The model under review builds one solid part; all positions refer to its coordinate system, in mm. A direction names the side the tool comes from. Round coordinates to 2 decimals unless told otherwise and drop trailing zeros. Write each loop counter-clockwise with the first axis right and the second up, starting at its lowest first coordinate (ties: lowest second). Pieces come first, ordered by that corner, then holes. Notation, with made-up numbers: (74.25, 74.25) -> (124.25, 74.25) arc R8 cw to (124.25, 82.25) -> close; hole circle Ø5 at (-2, 57). An arc over 180 degrees is marked (long way). Return JSON: item names as keys, results as strings. Group by question number.
1. Take a section at D-D, the plane y = -10. Write out the cut boundary in (x, z), then the cut area to 3 significant figures.
2. Take a section at A-A, the plane y = 18. Write out the cut boundary in (x, z), then the cut area to 3 significant figures.
3. For line 1 along Y through (x, z) = (-51.5, 8); line 2 along Y through (x, z) = (-27.5, 22); line 3 along X through (y, z) = (-12, 22), list the stretches that pass through material, from the lowest coordinate up. Write a range as from..to.
4. Mouldability with a two-part tool opening along Z and no side actions: class faces 1 (the flat face through (45.5, -58, 8)), 2 (the cylindrical face through (-20.03, 24.31, 6.08)), 3 (the cylindrical face through (50, -36, 8)), 4 (the cylindrical face through (-50, -34, 17)) as pulls with the +Z half, pulls with the -Z half, needs draft (parallel to the pull), parting line crosses it, or undercut.
5. Take a section at C-C, the plane x = 0. Write out the cut boundary in (y, z).
6. Clearance check with flat-ended pins moving along their axes: P1, Ø3, axis at x = 0, y = 56, coming from the -Z side; P2, Ø1.5, axis at x = -31.5, y = -42, coming from the +Z side; P3, Ø8, axis at x = 42, y = -38, coming from the +Z side. State where each tip first meets the part, or that it passes through.
7. Tool access review of faces 5 (the flat face through (-45.5, -58, 8)), 6 (the flat face through (-48.5, 30, 22)), 7 (the flat face through (0, -20, 6)): name each direction out of +Z, -Z, +X, -X, +Y, -Y from which nothing blocks a thin tool from reaching the whole face with its end or side.
8. Take a section at B-B, the plane z = 23. Write out the cut boundary in (x, y), then the cut area to 3 significant figures.
from build123d import *

# Parameters (mm, degrees)
SKETCH1_W           = 97
SKETCH1_H           = 130
BOSS_EXTRUDE1_DEPTH = 12
SKETCH9_R           = 32
CUT_EXTRUDE2_DEPTH  = 12
SKETCH11_W          = 109
SKETCH11_H          = 142
SKETCH11_W_2        = 97
SKETCH11_H_2        = 130
BOSS_EXTRUDE4_DEPTH = 32
SKETCH18_W          = 20
SKETCH18_H          = 60
BOSS_EXTRUDE5_DEPTH = 3
SKETCH14_R          = 15
CUT_EXTRUDE5_DEPTH  = 134.962681371
SKETCH20_W          = 91
SKETCH20_H          = 20
BOSS_EXTRUDE6_DEPTH = 4
SKETCH21_R          = 2
CUT_EXTRUDE6_DEPTH  = 9
SKETCH23_R          = 2
CUT_EXTRUDE7_DEPTH  = 6
BOSS_EXTRUDE7_START = -12
SKETCH26_R          = 32
SKETCH26_R_2        = 21
BOSS_EXTRUDE7_DEPTH = 12


with BuildPart() as part:
    # Sketch1 → Boss-Extrude1 (new body)
    with BuildSketch(Plane.XY):
        Rectangle(SKETCH1_W, SKETCH1_H)
    extrude(amount=BOSS_EXTRUDE1_DEPTH)

    # Sketch9 → Cut-Extrude2 (cut)
    with BuildSketch(Plane.XY.offset(12)):
        with Locations((0, 18)):
            Circle(SKETCH9_R)
    extrude(amount=-CUT_EXTRUDE2_DEPTH, mode=Mode.SUBTRACT)

    # Sketch11 → Boss-Extrude4 (add)
    with BuildSketch(Plane.XY):
        Rectangle(SKETCH11_W, SKETCH11_H)
        Rectangle(SKETCH11_W_2, SKETCH11_H_2, mode=Mode.SUBTRACT)
    extrude(amount=BOSS_EXTRUDE4_DEPTH)

    # Sketch18 → Boss-Extrude5 (add)
    with BuildSketch(Plane(origin=(-48.5, 0, 0), x_dir=(0, 0, -1), z_dir=(1, 0, 0))):
        with Locations((-22, -35)):
            Rectangle(SKETCH18_W, SKETCH18_H)
    boss_extrude5 = extrude(amount=BOSS_EXTRUDE5_DEPTH)

    # Mirror1: Boss-Extrude5 across plane
    add(boss_extrude5.mirror(Plane(origin=(0, 0, 0), x_dir=(0, 0, 1), z_dir=(1, 0, 0))))

    # Sketch14 → Cut-Extrude5 (cut, through all)
    with BuildSketch(Plane.ZY.offset(54.5)):
        with Locations((32, -34)):
            Circle(SKETCH14_R)
    extrude(amount=-CUT_EXTRUDE5_DEPTH, mode=Mode.SUBTRACT)

    # Sketch20 → Boss-Extrude6 (add)
    with BuildSketch(Plane(origin=(0, -65, 0), x_dir=(1, 0, 0), z_dir=(0, 1, 0))):
        with Locations((0, -22)):
            Rectangle(SKETCH20_W, SKETCH20_H)
    extrude(amount=BOSS_EXTRUDE6_DEPTH)

    # Sketch21 → Cut-Extrude6 (cut)
    with BuildSketch(Plane.ZY.offset(54.5)):
        with Locations((32, -10)):
            Circle(SKETCH21_R)
        with Locations((8, -10)):
            Circle(SKETCH21_R)
        with Locations((56, -10)):
            Circle(SKETCH21_R)
        with Locations((56, -58)):
            Circle(SKETCH21_R)
        with Locations((32, -58)):
            Circle(SKETCH21_R)
        with Locations(Location((8, -58, 0), (0, 0, 180))):
            Circle(SKETCH21_R)
        with Locations((8, -34)):
            Circle(SKETCH21_R)
    cut_extrude6 = extrude(amount=-CUT_EXTRUDE6_DEPTH, mode=Mode.SUBTRACT)

    # Mirror2: Cut-Extrude6 across plane
    add(cut_extrude6.mirror(Plane(origin=(0, 0, 0), x_dir=(0, 0, 1), z_dir=(1, 0, 0))), mode=Mode.SUBTRACT)

    # Sketch23 → Cut-Extrude7 (cut)
    with BuildSketch(Plane(origin=(0, 0, 0), x_dir=(-1, 0, 0), z_dir=(0, 0, -1))):
        with Locations((0, 56)):
            Circle(SKETCH23_R)
        with Locations((32.908965344, 37)):
            Circle(SKETCH23_R)
        with Locations((32.908965344, -1)):
            Circle(SKETCH23_R)
        with Locations((0, -20)):
            Circle(SKETCH23_R)
        with Locations((-32.908965344, -1)):
            Circle(SKETCH23_R)
        with Locations((-32.908965344, 37)):
            Circle(SKETCH23_R)
    extrude(amount=-CUT_EXTRUDE7_DEPTH, mode=Mode.SUBTRACT)

    # Sketch26 → Boss-Extrude7 (add)
    with BuildSketch(Plane(origin=(0, 0, 0), x_dir=(-1, 0, 0), z_dir=(0, 0, -1)).offset(BOSS_EXTRUDE7_START)):
        with Locations((0, 18)):
            Circle(SKETCH26_R)
        with Locations((0, 18)):
            Circle(SKETCH26_R_2, mode=Mode.SUBTRACT)
    extrude(amount=BOSS_EXTRUDE7_DEPTH)


solid = part.part
Output:
{
 "1": {"outline": "(-54.5, 0) -> (54.5, 0) -> (54.5, 6) -> (45.5, 6) -> (45.5, 10) -> (54.5, 10) -> (54.5, 30) -> (45.5, 30) -> (45.5, 12) -> (-45.5, 12) -> (-45.5, 30) -> (-54.5, 30) -> (-54.5, 10) -> (-45.5, 10) -> (-45.5, 6) -> (-54.5, 6) -> close", "area": "1,560 mm^2"},
 "2": {"outline": "(-54.5, 0) -> (-21, 0) -> (-21, 12) -> (-48.5, 12) -> (-48.5, 32) -> (-54.5, 32) -> close; (21, 0) -> (54.5, 0) -> (54.5, 32) -> (48.5, 32) -> (48.5, 12) -> (21, 12) -> close", "area": "1,040 mm^2"},
 "3": {"line 1": "y = -71..-60, -56..-36, -32..-12, -8..71", "line 2": "y = -71..-61, 65..71", "line 3": "x = -54.5..-45.5, 45.5..54.5"},
 "4": {"face 1": "undercut", "face 2": "needs draft", "face 3": "undercut", "face 4": "pulls with the +Z half"},
 "5": {"outline": "(-71, 0) -> (-22, 0) -> (-22, 6) -> (-18, 6) -> (-18, 0) -> (-3, 0) -> (-3, 12) -> (-61, 12) -> (-61, 32) -> (-71, 32) -> close; (39, 0) -> (54, 0) -> (54, 6) -> (58, 6) -> (58, 0) -> (71, 0) -> (71, 32) -> (65, 32) -> (65, 12) -> (39, 12) -> close"},
 "6": {"P1": "stops at z = 6", "P2": "stops at z = 12", "P3": "stops at z = 18.22"},
 "7": {"face 5": "-X", "face 6": "+Z", "face 7": "-Z"},
 "8": {"outline": "(-54.5, -71) -> (54.5, -71) -> (54.5, -46) -> (45.5, -46) -> (45.5, -61) -> (-45.5, -61) -> (-45.5, -46) -> (-54.5, -46) -> close; (-54.5, -22) -> (-45.5, -22) -> (-45.5, -5) -> (-48.5, -5) -> (-48.5, 65) -> (48.5, 65) -> (48.5, -5) -> (45.5, -5) -> (45.5, -22) -> (54.5, -22) -> (54.5, 71) -> (-54.5, 71) -> close", "area": "3,160 mm^2"}
}
